Drawing for the job (mm, zero at the part's lowest x, y, z). Give positions to 0.01 mm unless a question says otherwise; leave off trailing zeros. Loops run counter-clockwise (first coordinate to the right, second up) from the corner with the lowest first, then second, coordinate; pieces in that order, holes last. Notation, with made-up numbers: (20.5, -39.5) -> (75.5, -39.5) arc R26 cw to (75.5, -3.5) -> close; hole circle Ø9 at (65, 17.25). An arc over 180 degrees is marked (long way). Write item = value, one per line.
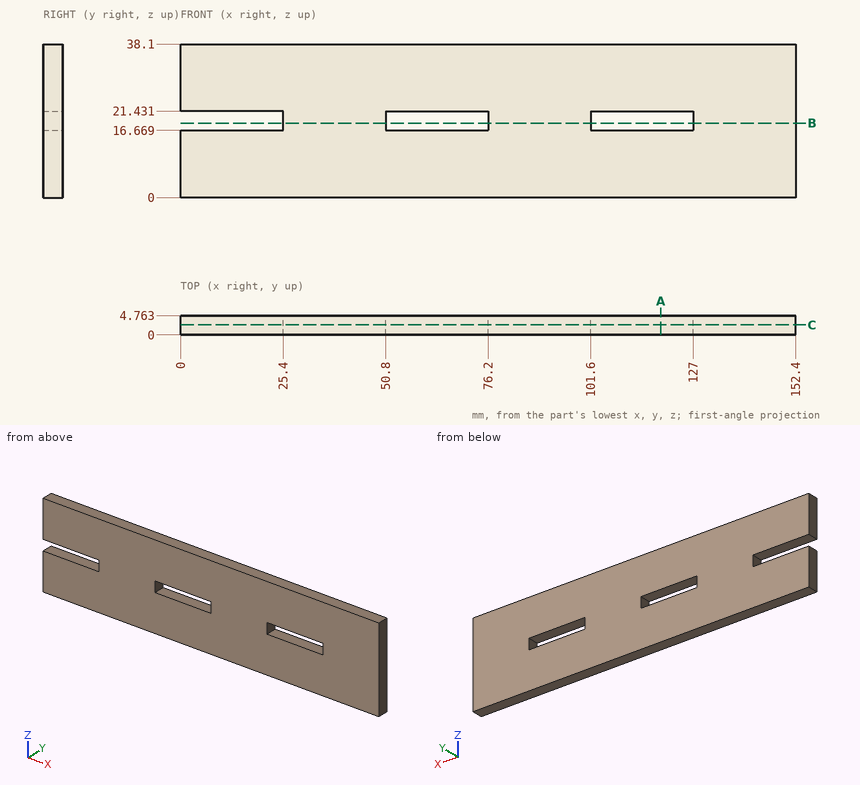
1) Drill centre lines: line 1 along X through (y, z) = (4.55, 20.5); line 2 along Z through (x, y) = (120.5, 1.8). Where is each one in solid material? Low to high. Write a range as [from, to].
Resolved:
line_1 = [25.4, 50.8], [76.2, 101.6], [127, 152.4]
line_2 = [0, 16.67], [21.43, 38.1]
2) Slice it at A-A, the plane x = 119. List the corners of the cut face in (y, z), and give its area (3 significant figures).
Resolved:
outline = (0, 0) -> (4.76, 0) -> (4.76, 16.67) -> (0, 16.67) -> close; (0, 21.43) -> (4.76, 21.43) -> (4.76, 38.1) -> (0, 38.1) -> close
area = 159 mm²
3) Drop a flat-ended pin along its axis: P1, Ø2.5, axis at y = 2, z = 19, coming from the -X side. Give the stop position or say it passes through.
Resolved:
P1 = 25.4
4) Slice it at C-C, the plane y = 2.5. List the corners of the cut face in (x, z), and give its area (3 significant figures).
Resolved:
outline = (0, 0) -> (152.4, 0) -> (152.4, 38.1) -> (0, 38.1) -> (0, 21.43) -> (25.4, 21.43) -> (25.4, 16.67) -> (0, 16.67) -> close; hole (50.8, 16.67) -> (76.2, 16.67) -> (76.2, 21.43) -> (50.8, 21.43) -> close; hole (101.6, 16.67) -> (127, 16.67) -> (127, 21.43) -> (101.6, 21.43) -> close
area = 5,440 mm²
5) Slice it at B-B, the plane z = 18.5. List the corners of the cut face in (x, y), and give its area (3 significant figures).
Resolved:
outline = (25.4, 0) -> (50.8, 0) -> (50.8, 4.76) -> (25.4, 4.76) -> close; (76.2, 0) -> (101.6, 0) -> (101.6, 4.76) -> (76.2, 4.76) -> close; (127, 0) -> (152.4, 0) -> (152.4, 4.76) -> (127, 4.76) -> close
area = 363 mm²
